Input: part model. Units: mm. Frame: model coordinates. A direction names the side the tool comes from. Round coordinates to 2 decimals unless told otherwise and drop trailing zeros. Order: outer loops, then holes, each group sorted by start corner. A loop starts at its lowest first (then second) coordinate and runs counter-clockwise, first axis right, second up. Notation, with made-up numbers: (-14, 31.25) -> (9, 31.25) arc R10 cw to (9, 37.25) -> close; hole circle Ø4 at (48.5, 55). An arc over 180 degrees is marked (long way). Use a Markdown table: item, result.
from build123d import *

# Parameters (mm, degrees)
F0_W     = 240.0041820114
F0_H     = 240.5
F0_R     = 2.75
F2_DEPTH = 7
F1_W     = 99.5
F1_H     = 99.5
F3_DEPTH = 7
F4_D     = 5.5
F4_DEPTH = 60
F4_TIP   = 1.6523667023
F5_DEPTH = 10
F7_D     = 6
F7_DEPTH = 2
F7_TIP   = 1.8025818571
F9_D     = 6
F9_DEPTH = 2
F9_TIP   = 1.8025818571


# Not quite as in the source:
# - a feature names something its author has since deleted; it is built from what else it names


with BuildPart() as f2:
    # F0 (on Top) → F2 (new body)
    with BuildSketch(Plane.XY):
        Rectangle(F0_W, F0_H)
        Polygon((-118, -60.5), (-94.8284271247, -60.5), (-37.3284271247, -118), (-118, -118), align=None, mode=Mode.SUBTRACT)
        Polygon((-69.8158430413, -58.5), (-118, -58.5), (-118, -1), (-92.2, -1), (-92.2, -22.25), (-67.7, -22.25), (-67.7, -1), (-12.3158430413, -1), align=None, mode=Mode.SUBTRACT)
        Polygon((118, -118), (-34.5, -118), (-92, -60.5), (118, -60.5), align=None, mode=Mode.SUBTRACT)
        with BuildLine():
            Line((118, -1), (118, -58.5))
            Line((118, -58.5), (-66.9874159165, -58.5))
            Line((-66.9874159165, -58.5), (-9.4874159165, -1))
            Line((-9.4874159165, -1), (-4.6435439053, -1))
            ThreePointArc((-4.6435439053, -1), (0, -4.75), (4.6435439053, -1))
            Line((4.6435439053, -1), (67.6999996539, -1))
            Line((67.6999996539, -1), (67.699995977, -22.25))
            Line((67.699995977, -22.25), (92.2, -22.25))
            Line((92.2, -22.25), (92.2, -1))
            Line((92.2, -1), (118, -1))
        make_face(mode=Mode.SUBTRACT)
        Polygon((-69.7, 20.25), (-69.7, 0), (-69.7, -20.25), (-90.2, -20.25), (-90.2, 0), (-90.2, 20.25), align=None, mode=Mode.SUBTRACT)
        with BuildLine():
            Line((-118.05, 1), (-118.05, 58.5))
            Line((-118.05, 58.5), (16.9895635103, 58.5))
            Line((16.9895635103, 58.5), (67.7, 7.7895635103))
            Line((67.7, 7.7895635103), (67.7, 1))
            Line((67.7, 1), (4.6435439053, 1))
            ThreePointArc((4.6435439053, 1), (0, 4.75), (-4.6435439053, 1))
            Line((-4.6435439053, 1), (-67.7, 1))
            Line((-67.7, 1), (-67.7, 22.25))
            Line((-67.7, 22.25), (-92.2, 22.25))
            Line((-92.2, 22.25), (-92.2, 1))
            Line((-92.2, 1), (-118.05, 1))
        make_face(mode=Mode.SUBTRACT)
        Polygon((-118, 60.5), (-118, 118), (-18.9642378869, 118), (-76.4642378869, 60.5), align=None, mode=Mode.SUBTRACT)
        Circle(F0_R, mode=Mode.SUBTRACT)
        Polygon((69.7, -20.25), (69.7, -2.25), (69.7, 20.25), (90.2, 20.25), (90.2, -2.25), (90.2, -20.25), align=None, mode=Mode.SUBTRACT)
        Polygon((67.7, 22.25), (67.7, 10.617990635), (19.817990635, 58.5), (118, 58.5), (118, 0.9999998737), (92.2, 0.9999998737), (92.2, 22.25), align=None, mode=Mode.SUBTRACT)
        Polygon((118, 118), (118, 60.5), (-73.6358107621, 60.5), (-16.1358107621, 118), align=None, mode=Mode.SUBTRACT)
        Polygon((-92, -60.5), (-34.5, -118), (118, -118), (118, -60.5), align=None)
        Polygon((-73.6358107621, 60.5), (118, 60.5), (118, 118), (-16.1358107621, 118), align=None)
        with BuildLine():
            Line((16.9895635103, 58.5), (-118.05, 58.5))
            Line((-118.05, 58.5), (-118.05, 1))
            Line((-118.05, 1), (-92.2, 1))
            Line((-92.2, 1), (-92.2, 22.25))
            Line((-92.2, 22.25), (-67.7, 22.25))
            Line((-67.7, 22.25), (-67.7, 1))
            Line((-67.7, 1), (-4.6435439053, 1))
            ThreePointArc((-4.6435439053, 1), (0, 4.75), (4.6435439053, 1))
            Line((4.6435439053, 1), (67.7, 1))
            Line((67.7, 1), (67.7, 7.7895635103))
            Line((67.7, 7.7895635103), (16.9895635103, 58.5))
        make_face()
        with BuildLine():
            Line((-66.9874159165, -58.5), (118, -58.5))
            Line((118, -58.5), (118, -1))
            Line((118, -1), (92.2, -1))
            Line((92.2, -1), (92.2, -22.25))
            Line((92.2, -22.25), (67.699995977, -22.25))
            Line((67.699995977, -22.25), (67.6999996539, -1))
            Line((67.6999996539, -1), (4.6435439053, -1))
            ThreePointArc((4.6435439053, -1), (0, -4.75), (-4.6435439053, -1))
            Line((-4.6435439053, -1), (-9.4874159165, -1))
            Line((-9.4874159165, -1), (-66.9874159165, -58.5))
        make_face()
        Polygon((-18.9642378869, 118), (-118, 118), (-118, 60.5), (-76.4642378869, 60.5), align=None)
        Polygon((-118, -1), (-118, -58.5), (-69.8158430413, -58.5), (-12.3158430413, -1), (-67.7, -1), (-67.7, -22.25), (-92.2, -22.25), (-92.2, -1), align=None)
        Polygon((19.817990635, 58.5), (67.7, 10.617990635), (67.7, 22.25), (92.2, 22.25), (92.2, 0.9999998737), (118, 0.9999998737), (118, 58.5), align=None)
        Polygon((-37.3284271247, -118), (-94.8284271247, -60.5), (-118, -60.5), (-118, -118), align=None)
    extrude(amount=F2_DEPTH)

    # F1 (on Top) → F3 (join)
    with BuildSketch(Plane.XY):
        Rectangle(F1_W, F1_H)
    extrude(amount=-F3_DEPTH)

    # F4
    with Locations(Plane.XY):
        with Locations((0, 0)):
            Hole(F4_D / 2, depth=F4_DEPTH)
            with Locations((0, 0, -(F4_DEPTH + F4_TIP / 2))):  # 118° drill point
                Cone(0, F4_D / 2, F4_TIP, mode=Mode.SUBTRACT)

    # F0 (on Top) → F5 (join)
    with BuildSketch(Plane.XY):
        Rectangle(F0_W, F0_H)
        Polygon((-118, -60.5), (-94.8284271247, -60.5), (-37.3284271247, -118), (-118, -118), align=None, mode=Mode.SUBTRACT)
        Polygon((-69.8158430413, -58.5), (-118, -58.5), (-118, -1), (-92.2, -1), (-92.2, -22.25), (-67.7, -22.25), (-67.7, -1), (-12.3158430413, -1), align=None, mode=Mode.SUBTRACT)
        Polygon((118, -118), (-34.5, -118), (-92, -60.5), (118, -60.5), align=None, mode=Mode.SUBTRACT)
        with BuildLine():
            Line((118, -1), (118, -58.5))
            Line((118, -58.5), (-66.9874159165, -58.5))
            Line((-66.9874159165, -58.5), (-9.4874159165, -1))
            Line((-9.4874159165, -1), (-4.6435439053, -1))
            ThreePointArc((-4.6435439053, -1), (0, -4.75), (4.6435439053, -1))
            Line((4.6435439053, -1), (67.6999996539, -1))
            Line((67.6999996539, -1), (67.699995977, -22.25))
            Line((67.699995977, -22.25), (92.2, -22.25))
            Line((92.2, -22.25), (92.2, -1))
            Line((92.2, -1), (118, -1))
        make_face(mode=Mode.SUBTRACT)
        Polygon((-69.7, 20.25), (-69.7, 0), (-69.7, -20.25), (-90.2, -20.25), (-90.2, 0), (-90.2, 20.25), align=None, mode=Mode.SUBTRACT)
        with BuildLine():
            Line((-118.05, 1), (-118.05, 58.5))
            Line((-118.05, 58.5), (16.9895635103, 58.5))
            Line((16.9895635103, 58.5), (67.7, 7.7895635103))
            Line((67.7, 7.7895635103), (67.7, 1))
            Line((67.7, 1), (4.6435439053, 1))
            ThreePointArc((4.6435439053, 1), (0, 4.75), (-4.6435439053, 1))
            Line((-4.6435439053, 1), (-67.7, 1))
            Line((-67.7, 1), (-67.7, 22.25))
            Line((-67.7, 22.25), (-92.2, 22.25))
            Line((-92.2, 22.25), (-92.2, 1))
            Line((-92.2, 1), (-118.05, 1))
        make_face(mode=Mode.SUBTRACT)
        Polygon((-118, 60.5), (-118, 118), (-18.9642378869, 118), (-76.4642378869, 60.5), align=None, mode=Mode.SUBTRACT)
        Circle(F0_R, mode=Mode.SUBTRACT)
        Polygon((69.7, -20.25), (69.7, -2.25), (69.7, 20.25), (90.2, 20.25), (90.2, -2.25), (90.2, -20.25), align=None, mode=Mode.SUBTRACT)
        Polygon((67.7, 22.25), (67.7, 10.617990635), (19.817990635, 58.5), (118, 58.5), (118, 0.9999998737), (92.2, 0.9999998737), (92.2, 22.25), align=None, mode=Mode.SUBTRACT)
        Polygon((118, 118), (118, 60.5), (-73.6358107621, 60.5), (-16.1358107621, 118), align=None, mode=Mode.SUBTRACT)
    extrude(amount=F5_DEPTH)

    # F7
    with Locations(Plane.XZ.offset(49.75)):
        with Locations((0, -3.5)):
            Hole(F7_D / 2, depth=F7_DEPTH)
            with Locations((0, 0, -(F7_DEPTH + F7_TIP / 2))):  # 118° drill point
                Cone(0, F7_D / 2, F7_TIP, mode=Mode.SUBTRACT)

    # F9
    with Locations(Plane(origin=(0, 49.75, 0), x_dir=(-1, 0, 0), z_dir=(0, 1, 0))):
        with Locations((0, -3.5)):
            Hole(F9_D / 2, depth=F9_DEPTH)
            with Locations((0, 0, -(F9_DEPTH + F9_TIP / 2))):  # 118° drill point
                Cone(0, F9_D / 2, F9_TIP, mode=Mode.SUBTRACT)


solid = f2.part
1) Cut plane C-C on y = -67.5. Return loops of the section in (x, z).
Answer key:
| item | result |
|---|---|
| outline | (-120, 0) -> (120, 0) -> (120, 10) -> (118, 10) -> (118, 7) -> (-85, 7) -> (-85, 10) -> (-87.83, 10) -> (-87.83, 7) -> (-118, 7) -> (-118, 10) -> (-120, 10) -> close |
2) Contact query for flat-ended pins moving along their axis: P1, Ø12, axis at x = -88, y = -82, coming from the -Z side; P2, Ø6, axis at y = -72.5, z = -4.5, coming from the -X side; P3, Ø3, axis at x = -5, z = -3, coming from the +Y side. Output: stop coordinate, or through.
Answer key:
| item | result |
|---|---|
| P1 | stops at z = 0 |
| P2 | passes through |
| P3 | stops at y = 49.75 |
3) Cut plane A-A on y = 53.5. Return loops of the section in (x, z).
Answer key:
| item | result |
|---|---|
| outline | (-120, 0) -> (120, 0) -> (120, 10) -> (118, 10) -> (118, 7) -> (24.82, 7) -> (24.82, 10) -> (21.99, 10) -> (21.99, 7) -> (-118.05, 7) -> (-118.05, 10) -> (-120, 10) -> close |
4) Set-up query: faces 1 (the face through (-38.64, -30.15, 8.48)), 2 (the face through (-2, 120.25, 5)), 3 (the face through (-80, 20.25, 5)), 4 (the face through (-49.75, -1, -3)), 5 (the face through (-0.7, 49.75, -6.6)). Return all of +Z, -Z, +X, -X, +Y, -Y with unobstructed straight access to the full face (end or side cutting, diameter ignored); none if empty.
Answer key:
| item | result |
|---|---|
| face 1 | +Z |
| face 2 | +Z, -Z, +X, -X, +Y |
| face 3 | +Z, -Z |
| face 4 | -Z, -X, +Y, -Y |
| face 5 | -Z, +X, -X, +Y |
5) Draft query along Z for faces 6 (the face through (-18.3, 0.6, 10)), 7 (the face through (-2, -120.25, 5)), 8 (the face through (0.497, -46.26, -3.344)), 9 (the face through (-0.497, 46.26, -3.344)). Return one class per face: released by +Z, released by -Z, zero draft, split by the parting line, or undercut.
Answer key:
| item | result |
|---|---|
| face 6 | released by +Z |
| face 7 | zero draft |
| face 8 | undercut |
| face 9 | undercut |
6) Cut plane B-B on y = -38. Return loops of the section in (x, z), and give its area (3 significant figures).
Answer key:
| item | result |
|---|---|
| outline | (-120, 0) -> (-49.75, 0) -> (-49.75, -7) -> (49.75, -7) -> (49.75, 0) -> (120, 0) -> (120, 10) -> (118, 10) -> (118, 7) -> (-46.49, 7) -> (-46.49, 10) -> (-49.32, 10) -> (-49.32, 7) -> (-118, 7) -> (-118, 10) -> (-120, 10) -> close |
| area | 2,400 mm^2 |
7) Ray query, probe 1 along X at (y, z) = (0, 8.95); probe 2 along X at (y, z) = (-48.55, -3.5); probe 3 along X at (y, z) = (-14, 1.5). Return the intervals inside material, ascending.
Answer key:
| item | result |
|---|---|
| probe 1 | x = -120 to -90.2, -69.7 to -2.75, 2.75 to 69.7, 90.2 to 120 |
| probe 2 | x = -49.75 to -3, 3 to 49.75 |
| probe 3 | x = -120 to -90.2, -69.7 to 69.7, 90.2 to 120 |
